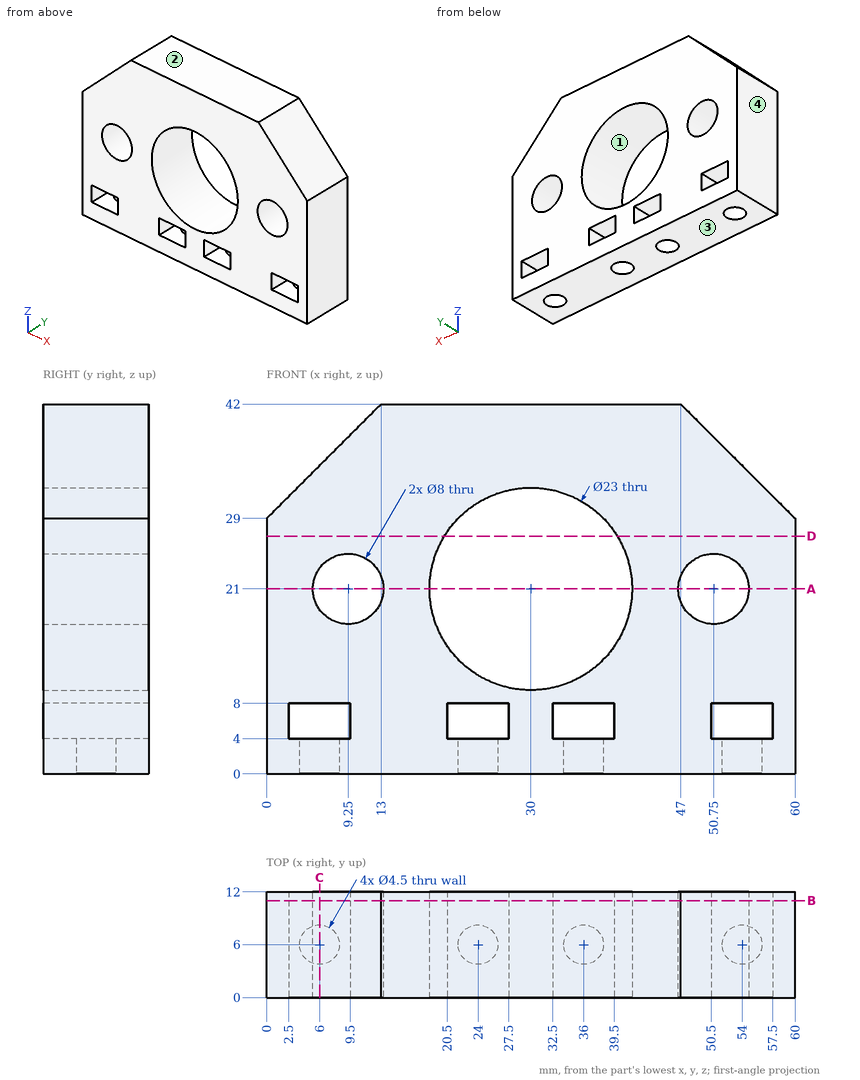
Part print with two shaded views. Sizes in mm from the minimum x, y, z corner. Coordinates: 2 decimals unless noted, no trailing zeros. Write each loop counter-clockwise with the first axis right and the second up, starting at its lowest first coordinate (ties: lowest second). Pieces come first, ordered by that corner, then holes.
1. Pull direction Z, two halves, no side cores. Call the marked faces 1, 2, 3 and 4: released by +Z, released by -Z, zero draft, split by the parting line, or undercut.
Answer block:
face 1: undercut
face 2: released by +Z
face 3: released by -Z
face 4: zero draft
2. Band-saw the part on B-B, the plane y = 11. Give the cut face in (x, z), and give its area (3 significant figures).
Answer block:
outline: (0, 0) - (60, 0) - (60, 29) - (47, 42) - (13, 42) - (0, 29) - close; hole (2.5, 4) - (9.5, 4) - (9.5, 8) - (2.5, 8) - close; hole circle Ø8 at (9.25, 21); hole circle Ø23 at (30, 21); hole (20.5, 4) - (27.5, 4) - (27.5, 8) - (20.5, 8) - close; hole (32.5, 4) - (39.5, 4) - (39.5, 8) - (32.5, 8) - close; hole circle Ø8 at (50.75, 21); hole (50.5, 4) - (57.5, 4) - (57.5, 8) - (50.5, 8) - close
area: 1,720 mm2
3. Band-saw the part on A-A, the plane z = 21. Give the cut face in (x, y).
Answer block:
outline: (0, 0) - (5.25, 0) - (5.25, 12) - (0, 12) - close; (13.25, 0) - (18.5, 0) - (18.5, 12) - (13.25, 12) - close; (41.5, 0) - (46.75, 0) - (46.75, 12) - (41.5, 12) - close; (54.75, 0) - (60, 0) - (60, 12) - (54.75, 12) - close
4. Drill centre lines: probe 1 along X at (y, z) = (2.5, 4.5); probe 2 along X at (y, z) = (5.5, 21); probe 3 along Z at (x, y) = (50.75, 8). Where is each one in solid material? Low to high.
Answer block:
probe 1: x = 0 to 2.5, 9.5 to 20.5, 27.5 to 32.5, 39.5 to 50.5, 57.5 to 60
probe 2: x = 0 to 5.25, 13.25 to 18.5, 41.5 to 46.75, 54.75 to 60
probe 3: z = 0 to 4, 8 to 17, 25 to 38.25
5. Band-saw the part on D-D, the plane z = 27. Give the cut face in (x, y).
Answer block:
outline: (0, 0) - (20.19, 0) - (20.19, 12) - (0, 12) - close; (39.81, 0) - (60, 0) - (60, 12) - (39.81, 12) - close
6. Drop flat-ended pins along their axis: pin 1 (3 mm diameter, centred on y = 3, z = 34.5, fed in from +X); pin 2 (2 mm diameter, centred on x = 10.5, y = 9, fed in from +Z); pin 3 (2 mm diameter, centred on x = 36.5, y = 7, fed in from -Z). Give the stop position or say it passes through.
Answer block:
pin 1: stops at x = 56
pin 2: stops at z = 40.5
pin 3: stops at z = 8
7. Band-saw the part on C-C, the plane x = 6. Give the cut face in (y, z).
Answer block:
outline: (0, 0) - (3.75, 0) - (3.75, 4) - (0, 4) - close; (0, 8) - (12, 8) - (12, 18.67) - (0, 18.67) - close; (0, 23.33) - (12, 23.33) - (12, 35) - (0, 35) - close; (8.25, 0) - (12, 0) - (12, 4) - (8.25, 4) - close
